```python
from build123d import *

# Parameters (mm, degrees)
SKETCH1_W                = 20
SKETCH1_H                = 33
SKETCH1_W_2              = 1010
BOSS_EXTRUDE1_DEPTH      = 10.5
CUT_EXTRUDE1_START       = 26
CUT_EXTRUDE1_DEPTH       = 21
F_9_0_9_DIAMETER_HOLE1_D = 9


with BuildPart() as part:
    # Sketch1 → Boss-Extrude1 (new, symmetric)
    # profile 1 of 5: a face of its own
    with BuildSketch(Plane.XY):
        with Locations((1020, 16.5)):
            Rectangle(SKETCH1_W, SKETCH1_H)
        with BuildLine():
            Line((1025.5, 20.5), (1025.5, 12.5))
            ThreePointArc((1025.5, 12.5), (1020, 7), (1014.5, 12.5))
            Line((1014.5, 12.5), (1014.5, 20.5))
            ThreePointArc((1014.5, 20.5), (1020, 26), (1025.5, 20.5))
        make_face(mode=Mode.SUBTRACT)
    # profile 2 of 5: a face of its own
    with BuildSketch(Plane.XY):
        with BuildLine():
            ThreePointArc((1025.5, 12.5), (1020, 7), (1014.5, 12.5))
            Line((1014.5, 12.5), (1014.5, 20.5))
            ThreePointArc((1014.5, 20.5), (1020, 26), (1025.5, 20.5))
            Line((1025.5, 20.5), (1025.5, 12.5))
        make_face()
        with BuildLine():
            Line((1023, 20.5), (1023, 12.5))
            ThreePointArc((1023, 12.5), (1020, 9.5), (1017, 12.5))
            Line((1017, 12.5), (1017, 20.5))
            ThreePointArc((1017, 20.5), (1020, 23.5), (1023, 20.5))
        make_face(mode=Mode.SUBTRACT)
    # profile 3 of 5: a face of its own
    with BuildSketch(Plane.XY):
        with Locations((505, 16.5)):
            Rectangle(SKETCH1_W_2, SKETCH1_H)
    # profile 4 of 5: a face of its own
    with BuildSketch(Plane.XY):
        with Locations((-10, 16.5)):
            Rectangle(SKETCH1_W, SKETCH1_H)
        with BuildLine():
            ThreePointArc((-4.5, 20.5), (-10, 26), (-15.5, 20.5))
            Line((-15.5, 20.5), (-15.5, 12.5))
            ThreePointArc((-15.5, 12.5), (-10, 7), (-4.5, 12.5))
            Line((-4.5, 12.5), (-4.5, 20.5))
        make_face(mode=Mode.SUBTRACT)
    # profile 5 of 5: a face of its own
    with BuildSketch(Plane.XY):
        with BuildLine():
            Line((-4.5, 20.5), (-4.5, 12.5))
            ThreePointArc((-4.5, 12.5), (-10, 7), (-15.5, 12.5))
            Line((-15.5, 12.5), (-15.5, 20.5))
            ThreePointArc((-15.5, 20.5), (-10, 26), (-4.5, 20.5))
        make_face()
        with BuildLine():
            ThreePointArc((-13, 12.5), (-10, 9.5), (-7, 12.5))
            Line((-7, 12.5), (-7, 20.5))
            ThreePointArc((-7, 20.5), (-10, 23.5), (-13, 20.5))
            Line((-13, 20.5), (-13, 12.5))
        make_face(mode=Mode.SUBTRACT)
    extrude(amount=BOSS_EXTRUDE1_DEPTH, both=True)

    # Sketch1_3 → Cut-Extrude1 (cut)
    # profile 1 of 2: a face of its own
    with BuildSketch(Plane.XY.offset(CUT_EXTRUDE1_START)):
        with BuildLine():
            Line((-4.5, 20.5), (-4.5, 12.5))
            ThreePointArc((-4.5, 12.5), (-10, 7), (-15.5, 12.5))
            Line((-15.5, 12.5), (-15.5, 20.5))
            ThreePointArc((-15.5, 20.5), (-10, 26), (-4.5, 20.5))
        make_face()
        with BuildLine():
            ThreePointArc((-13, 12.5), (-10, 9.5), (-7, 12.5))
            Line((-7, 12.5), (-7, 20.5))
            ThreePointArc((-7, 20.5), (-10, 23.5), (-13, 20.5))
            Line((-13, 20.5), (-13, 12.5))
        make_face(mode=Mode.SUBTRACT)
    # profile 2 of 2: a face of its own
    with BuildSketch(Plane.XY.offset(CUT_EXTRUDE1_START)):
        with BuildLine():
            ThreePointArc((1025.5, 12.5), (1020, 7), (1014.5, 12.5))
            Line((1014.5, 12.5), (1014.5, 20.5))
            ThreePointArc((1014.5, 20.5), (1020, 26), (1025.5, 20.5))
            Line((1025.5, 20.5), (1025.5, 12.5))
        make_face()
        with BuildLine():
            Line((1023, 20.5), (1023, 12.5))
            ThreePointArc((1023, 12.5), (1020, 9.5), (1017, 12.5))
            Line((1017, 12.5), (1017, 20.5))
            ThreePointArc((1017, 20.5), (1020, 23.5), (1023, 20.5))
        make_face(mode=Mode.SUBTRACT)
    cut_extrude1 = extrude(amount=-CUT_EXTRUDE1_DEPTH, mode=Mode.SUBTRACT)

    # Mirror1: Cut-Extrude1 across plane
    add(cut_extrude1.mirror(Plane.XY), mode=Mode.SUBTRACT)

    # 9.0 _9_ Diameter Hole1 (through all)
    with Locations(Plane(origin=(0, 33, 0), x_dir=(1, 0, 0), z_dir=(0, 1, 0))):
        with Locations((-10, 0), (1020, 0)):
            Hole(F_9_0_9_DIAMETER_HOLE1_D / 2)


solid = part.part
```
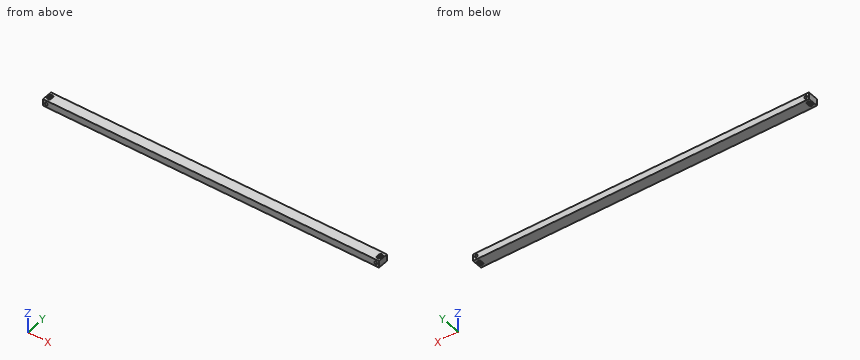
Geometry: final body of the model. Coordinates: model frame, mm. Give positions to 0.01 mm unless a question says otherwise; leave off trailing zeros. Loops run counter-clockwise (first coordinate to the right, second up) from the corner with the lowest first, then second, coordinate; pieces in that order, holes last. Notation, with made-up numbers: (53.25, 45) -> (91.25, 45) arc R38 cw to (91.25, 83) -> close; hole circle Ø7 at (6, 44.25). An arc over 180 degrees is marked (long way). Use one line per item in the form item = value.
Item 1: Line query: probe 1 along X at (y, z) = (20, 1.25); probe 2 along X at (y, z) = (13, 9.5); probe 3 along Z at (x, y) = (-10, 8). Output: solid intervals per line, ascending.
A:
probe_1 = -20 to -14.32, -5.68 to 1015.68, 1024.32 to 1030
probe_2 = -20 to -15.5, -4.5 to 1014.5, 1025.5 to 1030
probe_3 = -5 to -4.5, 4.5 to 5
Item 2: Section query A-A on z = 0. Output: boundary loops of the cut face in (x, y), and give its area (3 significant figures).
A:
outline = (-20, 0) -> (-14.5, 0) -> (-14.5, 33) -> (-20, 33) -> close; (-5.5, 0) -> (1015.5, 0) -> (1015.5, 33) -> (-5.5, 33) -> close; (1024.5, 0) -> (1030, 0) -> (1030, 33) -> (1024.5, 33) -> close
area = 34,100 mm^2
Item 3: Pin query (flat end, axial travel): P1, Ø3.5, axis at x = -12.5, y = 15.5, coming from the +Z side. Return the tip coordinate at first contact, or that it passes through.
A:
P1 = 5
